Check sheet for the modelled part. Datum: model origin and axes. Units: mm. Round coordinates to 2 decimals unless told otherwise and drop trailing zeros. Write each loop counter-clockwise with the first axis right and the second up, starting at its lowest first coordinate (ties: lowest second). Pieces come first, ordered by that corner, then holes. Notation, with made-up numbers: (73, -5.5) -> (122, -5.5) arc R19 ccw to (122, 22.5) -> close; hole circle Ø10 at (-16.5, -9.75). An arc over 180 degrees is marked (long way). Write item = value, one per line.
from build123d import *

# Parameters (mm, degrees)
SKETCH1_W            = 80
SKETCH1_H            = 15
BOSS_EXTRUDE1_DEPTH  = 13
M5_CLEARANCE_HOLE1_D = 5.3
FILLET1_R            = 5


with BuildPart() as part:
    # Sketch1 → Boss-Extrude1 (new body)
    with BuildSketch(Plane(origin=(0, 0, 0), x_dir=(1, 0, 0), z_dir=(0, 1, 0))):
        Rectangle(SKETCH1_W, SKETCH1_H)
    extrude(amount=-BOSS_EXTRUDE1_DEPTH)

    # M5 Clearance Hole1 (through all)
    with Locations(Plane(origin=(-32.5, 0, 0), x_dir=(0, 0, 1), z_dir=(0, 1, 0))):
        with Locations((0, 0), (0, 32.5), (0, 65)):
            Hole(M5_CLEARANCE_HOLE1_D / 2)

    # Fillet1
    fillet1_edges = [part.edges().sort_by_distance(p)[0] for p in [
        (-40, -6.5, -7.5),
        (40, -6.5, -7.5),
        (40, -6.5, 7.5),
        (-40, -6.5, 7.5),
    ]]
    fillet(fillet1_edges, radius=FILLET1_R)


solid = part.part
(1) Material ranges on L1, parallel to X at y = -10.25, z = 0; L2, parallel to X at y = -8.5, z = -2.25; L3, parallel to Z at x = -34, y = -6.25, recorded low to high. Write a range as [from, to].
Worked answers:
L1 = [-40, -35.15], [-29.85, -2.65], [2.65, 29.85], [35.15, 40]
L2 = [-40, -33.9], [-31.1, -1.4], [1.4, 31.1], [33.9, 40]
L3 = [-7.5, -2.18], [2.18, 7.5]
(2) Sectioned sample at A-A on x = 0. Enter the section's corners in (y, z).
Worked answers:
outline = (-13, -7.5) -> (0, -7.5) -> (0, -2.65) -> (-13, -2.65) -> close; (-13, 2.65) -> (0, 2.65) -> (0, 7.5) -> (-13, 7.5) -> close
(3) Release check for a two-part mould opening along X. For faces 1 (the cylindrical face through (35.13, -6.59, 0.34)), 2 (the cylindrical face through (38.5, -6.59, -6.07)), 3 (the flat face through (0, -6, 7.5)) record: pulls with the +X half, pulls with the -X half, needs draft (parallel to the pull), parting line crosses it, or undercut.
Worked answers:
face_1 = undercut
face_2 = pulls with the +X half
face_3 = needs draft
(4) Go/stop test with a flat-tipped pin: P1, Ø3, axis at x = 0, z = 0, coming from the +Y side. Record where the tip stops, or that it passes through.
Worked answers:
P1 = through
(5) Sectioned sample at B-B on y = -8.75. Enter the section's corners in (x, z), then the cut area to 3 significant figures.
Worked answers:
outline = (-40, -2.5) arc R5 ccw to (-35, -7.5) -> (35, -7.5) arc R5 ccw to (40, -2.5) -> (40, 2.5) arc R5 ccw to (35, 7.5) -> (-35, 7.5) arc R5 ccw to (-40, 2.5) -> close; hole circle Ø5.3 at (-32.5, 0); hole circle Ø5.3 at (0, 0); hole circle Ø5.3 at (32.5, 0)
area = 1,110 mm²
